```python
from build123d import *

# Parameters (mm, degrees)
SKETCH1_W           = 20
SKETCH1_H           = 15
BOSS_EXTRUDE1_DEPTH = 3.5
CUT_EXTRUDE1_DEPTH  = 1
CUT_EXTRUDE2_REACH  = 14.748
SKETCH3_W           = 4.5
SKETCH3_H           = 0.8
FILLET1_R           = 4
SKETCH4_W           = 4.5
SKETCH4_H           = 7.1
CUT_EXTRUDE3_DEPTH  = 0.4
FILLET2_R           = 1
BOSS_EXTRUDE2_START = 5
BOSS_EXTRUDE2_DEPTH = 5
FILLET3_R           = 1


with BuildPart() as part:
    # Sketch1 → Boss-Extrude1 (new body)
    with BuildSketch(Plane(origin=(0, 0, 0), x_dir=(1, 0, 0), z_dir=(0, 1, 0))):
        Rectangle(SKETCH1_W, SKETCH1_H)
    extrude(amount=BOSS_EXTRUDE1_DEPTH)

    # Sketch2 → Cut-Extrude1 (cut)
    with BuildSketch(Plane(origin=(0, 3.5, 0), x_dir=(1, 0, 0), z_dir=(0, 1, 0))):
        with BuildLine():
            Line((-2.65, -1.29614814), (-2.65, 1.29614814))
            ThreePointArc((-2.65, 1.29614814), (2.95, 0), (-2.65, -1.29614814))
        make_face()
    extrude(amount=-CUT_EXTRUDE1_DEPTH, mode=Mode.SUBTRACT)

    # Sketch3 → Cut-Extrude2 (cut, up to next)
    with BuildSketch(Plane(origin=(0, 2.5, 0), x_dir=(1, 0, 0), z_dir=(0, 1, 0)), mode=Mode.PRIVATE) as cut_extrude2_sk1:
        Rectangle(SKETCH3_W, SKETCH3_H)
    cut_extrude2_tool1 = extrude(cut_extrude2_sk1.sketch, amount=-CUT_EXTRUDE2_REACH, mode=Mode.PRIVATE) & part.part
    add(cut_extrude2_tool1.solids().sort_by_distance((0, 2.5, 0))[0], mode=Mode.SUBTRACT)

    # Fillet1
    fillet1_edges = [part.edges().sort_by_distance(p)[0] for p in [
        (-10, 1.75, -7.5),
        (10, 1.75, -7.5),
        (10, 1.75, 7.5),
        (-10, 1.75, 7.5),
    ]]
    fillet(fillet1_edges, radius=FILLET1_R)

    # Sketch4 → Cut-Extrude3 (cut)
    with BuildSketch(Plane.XZ):
        with Locations((0, -3.95)):
            Rectangle(SKETCH4_W, SKETCH4_H)
    extrude(amount=-CUT_EXTRUDE3_DEPTH, mode=Mode.SUBTRACT)

    # Fillet2
    fillet2_edges = [part.edges().sort_by_distance(p)[0] for p in [
        (0, 0.4, -0.4),
    ]]
    fillet(fillet2_edges, radius=FILLET2_R)

    # Sketch5 → Boss-Extrude2 (add)
    with BuildSketch(Plane(origin=(0, 3.5, 0), x_dir=(1, 0, 0), z_dir=(0, 1, 0)).offset(BOSS_EXTRUDE2_START)):
        with BuildLine():
            Line((-5, 7.5), (-5, -7.5))
            Line((-5, -7.5), (-6, -7.5))
            ThreePointArc((-6, -7.5), (-8.828427125, -6.328427125), (-10, -3.5))
            Line((-10, -3.5), (-10, 3.5))
            ThreePointArc((-10, 3.5), (-8.828427125, 6.328427125), (-6, 7.5))
            Line((-6, 7.5), (-5, 7.5))
        make_face()
        with BuildLine():
            Line((5, 7.5), (5, -7.5))
            Line((5, -7.5), (6, -7.5))
            ThreePointArc((6, -7.5), (8.828427125, -6.328427125), (10, -3.5))
            Line((10, -3.5), (10, 3.5))
            ThreePointArc((10, 3.5), (8.828427125, 6.328427125), (6, 7.5))
            Line((6, 7.5), (5, 7.5))
        make_face()
    extrude(amount=-BOSS_EXTRUDE2_DEPTH)

    # Fillet3
    fillet3_edges = [part.edges().sort_by_distance(p)[0] for p in [
        (5, 6, -7.5),
        (5, 6, 7.5),
        (-5, 6, -7.5),
        (-5, 6, 7.5),
    ]]
    fillet(fillet3_edges, radius=FILLET3_R - 0.0001)  # a hair under: the kernel refuses the full size


solid = part.part
```
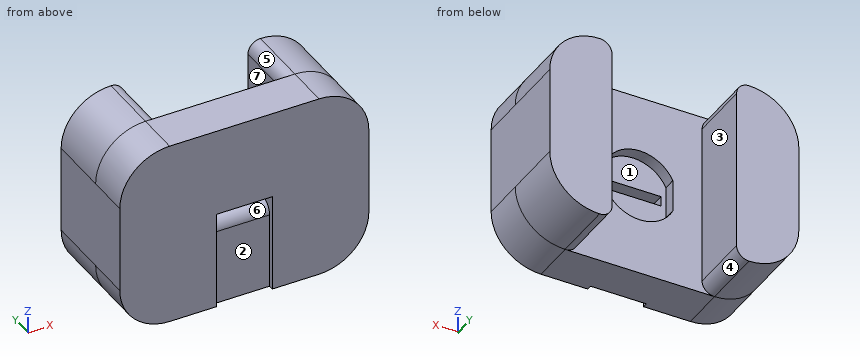
Build history of the part. All positions in model axes, mm. Face numbers are marked on the shaded views. A direction names the side the tool comes from. Give positions to 0.01 mm unless a question says otherwise; leave off trailing zeros. Order: outer loops, then holes, each group sorted by start corner. A loop starts at its lowest first (then second) coordinate and runs counter-clockwise, first axis right, second up. Notation, with made-up numbers: M 4.25,-4.75 L 40.25,-4.75 A23 ccw 40.25,9.25 Z; hole C 35.5,-8 d8. An arc over 180 degrees is marked long. Return JSON: item names as keys, results as strings.
Q1. Wall check: probe 1 along X at (y, z) = (7.75, -2.5); probe 2 along Z at (x, y) = (0, 3); probe 3 along Y at (x, z) = (-1.5, -5.5). Give the ranges that are in metal, low to high. Write a range as from..to.
Answer list:
{"probe 1": "x = -10..-5, 5..10", "probe 2": "z = -7.5..-2.95, 2.95..7.5", "probe 3": "y = 0.4..3.5"}
Q2. 3-axis set-ups, long thin cutter, end or side, ignore diameter. For the marked faces 1, 2 and 3: which of +Z, -Z, +X, -X, +Y, -Y reach the whole face in a straight line?
Answer list:
{"face 1": "+Y", "face 2": "-Z, -Y", "face 3": "+Z, -Z, +Y"}
Q3. Band-saw the part on B-B (y = 2.75). Give the cut face in (x, z).
Answer list:
{"outline": "M -10,-3.5 A4 ccw -6,-7.5 L 6,-7.5 A4 ccw 10,-3.5 L 10,3.5 A4 ccw 6,7.5 L -6,7.5 A4 ccw -10,3.5 Z; hole M -2.65,-1.3 A2.95 ccw long -2.65,1.3 Z"}
Q4. Band-saw the part on D-D (z = 2.25). Give the cut face in (x, y), then the cut area to 3 significant figures.
Answer list:
{"outline": "M -10,0 L 10,0 L 10,8.5 L 5,8.5 L 5,3.5 L 1.91,3.5 L 1.91,2.5 L -1.91,2.5 L -1.91,3.5 L -5,3.5 L -5,8.5 L -10,8.5 Z", "area": "116 mm^2"}
Q5. Band-saw the part on A-A (z = 0). Give the cut face in (x, y), then the cut area to 3 significant figures.
Answer list:
{"outline": "M -10,0 L -2.25,0 L -2.25,2.5 L -2.65,2.5 L -2.65,3.5 L -5,3.5 L -5,8.5 L -10,8.5 Z; M 2.25,0 L 10,0 L 10,8.5 L 5,8.5 L 5,3.5 L 2.95,3.5 L 2.95,2.5 L 2.25,2.5 Z", "area": "103 mm^2"}
Q6. Flat gauge pins, fed straight in: pin 1 (6 mm diameter, centred on x = 4.5, z = 1.5, fed in from +Y); pin 2 (2 mm diameter, centred on x = 0.5, z = -5, fed in from -Y); pin 3 (3 mm diameter, centred on x = -0.5, z = 1, fed in from +Y); pin 4 (6 mm diameter, centred on x = -1, z = 3, fed in from +Y). Where does each tip first touch, or does it go through?
Answer list:
{"pin 1": "stops at y = 8.5", "pin 2": "stops at y = 0.4", "pin 3": "stops at y = 2.5", "pin 4": "stops at y = 3.5"}
Q7. Band-saw the part on C-C (x = -1.5). Give the cut face in (y, z).
Answer list:
{"outline": "M 0,0.4 L 2.5,0.4 L 2.5,2.54 L 3.5,2.54 L 3.5,7.5 L 0,7.5 Z; M 0.4,-7.5 L 3.5,-7.5 L 3.5,-2.54 L 2.5,-2.54 L 2.5,-0.4 L 1.4,-0.4 A1 ccw 0.4,-1.4 Z"}
Q8. Two-plate mould, pull along Z, no slides. Class the marked faces 4, 5, 6 and 7: pulls with the +Z half, pulls with the -Z half, needs draft (parallel to the pull), parting line crosses it, or undercut.
Answer list:
{"face 4": "pulls with the -Z half", "face 5": "pulls with the +Z half", "face 6": "undercut", "face 7": "needs draft"}
